Input: part model. Units: mm. Frame: model coordinates. A direction names the side the tool comes from. Coordinates: 2 decimals unless noted, no trailing zeros. Write each loop counter-clockwise with the first axis right and the second up, starting at its lowest first coordinate (ties: lowest second). Pieces come first, ordered by that corner, then holes.
1) Section query D-D (x = -7). Output: boundary loops of the cut face in (y, z).
2) Section query C-C (y = 3.75). Output: boundary loops of the cut face in (x, z).
3) Pin query (flat end, axial travel): pin 1 Ø2.5 at (x, z) = (0, 0) entering from -Y; pin 2 Ø2 at (x, y) = (-7, 1) entering from -Z; pin 3 Ø1.5 at (y, z) = (2.5, 7.5) entering from +X; pin 4 Ø4 at (x, z) = (0, 7) entering from +Y. Return the tip coordinate at first contact, or that it passes through.
4) Section query B-B (z = -7). Output: boundary loops of the cut face in (x, y).
5) Section query A-A (x = 0). Output: boundary loops of the cut face in (y, z).
6) Set-up query: faces 4 (the cylindrical face through (5.536, 0.986, -0.325)), 5 (the flat face through (-2.1, 2, 4.3)). Return all of +Z, -Z, +X, -X, +Y, -Y with unobstructed straight access to the full face (end or side cutting, diameter ignored); none if empty.
7) Draft query along Z for faces 1 (the cylindrical face through (-8.464, 0.986, -0.325)), 2 (the cylindrical face through (-9.76, 0.99, -2.17)), 3 (the flat face through (-2, 4.5, 2)). Return one class per face: pulls with the +Z half, pulls with the -Z half, needs draft (parallel to the pull), parting line crosses it, or undercut.
8) Line query: L1, parallel to X at y = 0.55, z = 0; L2, parallel to X at y = 1.25, z = 0; L3, parallel to Y at x = -9, z = -0.25. Output: solid intervals per line, ascending.
from build123d import *

# Parameters (mm, degrees)
SKETCH_1_R          = 10
SKETCH_1_R_2        = 1.5
EXTRUDE_1_DEPTH     = 2
SKETCH_2_R          = 4.5
EXTRUDE_2_DEPTH     = 2.5
SKETCH_3_R          = 1.5
CUT_EXTRUDE_1_DEPTH = 15.84082208
SKETCH_4_R          = 2.5
CUT_EXTRUDE_2_DEPTH = 3.5


with BuildPart() as part:
    # 草图1 → 凸台-拉伸1 (new body)
    with BuildSketch(Plane(origin=(0, 0, 0), x_dir=(1, 0, 0), z_dir=(0, 1, 0))):
        with Locations(Location((0, 0, 0), (0, 0, 270))):
            Circle(SKETCH_1_R)
        with Locations(Location((0, 7, 0), (0, 0, 270))):
            Circle(SKETCH_1_R_2, mode=Mode.SUBTRACT)
        with Locations(Location((7, 0, 0), (0, 0, 270))):
            Circle(SKETCH_1_R_2, mode=Mode.SUBTRACT)
        with Locations(Location((0, -7, 0), (0, 0, 270))):
            Circle(SKETCH_1_R_2, mode=Mode.SUBTRACT)
        with Locations(Location((-7, 0, 0), (0, 0, 270))):
            Circle(SKETCH_1_R_2, mode=Mode.SUBTRACT)
    extrude(amount=EXTRUDE_1_DEPTH)

    # 草图2 → 凸台-拉伸2 (add)
    with BuildSketch(Plane(origin=(0, 2, 0), x_dir=(1, 0, 0), z_dir=(0, 1, 0))):
        with Locations(Location((0, 0, 0), (0, 0, 270))):
            Circle(SKETCH_2_R)
    extrude(amount=EXTRUDE_2_DEPTH)

    # 草图3 → 切除-拉伸1 (cut, through all)
    with BuildSketch(Plane(origin=(0, 4.5, 0), x_dir=(1, 0, 0), z_dir=(0, 1, 0))):
        with Locations(Location((0, 0, 0), (0, 0, 270))):
            Circle(SKETCH_3_R)
    extrude(amount=-CUT_EXTRUDE_1_DEPTH, mode=Mode.SUBTRACT)

    # 草图4 → 切除-拉伸2 (cut)
    with BuildSketch(Plane(origin=(0, 4.5, 0), x_dir=(1, 0, 0), z_dir=(0, 1, 0))):
        with Locations(Location((0, 0, 0), (0, 0, 270))):
            Circle(SKETCH_4_R)
    extrude(amount=-CUT_EXTRUDE_2_DEPTH, mode=Mode.SUBTRACT)


solid = part.part
Answer:
1. outline: (0, -7.14) - (2, -7.14) - (2, -1.5) - (0, -1.5) - close; (0, 1.5) - (2, 1.5) - (2, 7.14) - (0, 7.14) - close
2. outline: circle Ø9 at (0, 0); hole circle Ø5 at (0, 0)
3. pin 1: passes through
3. pin 2: stops at z = -8
3. pin 3: stops at x = 7.2
3. pin 4: stops at y = 2
4. outline: (-7.14, 0) - (-1.5, 0) - (-1.5, 2) - (-7.14, 2) - close; (1.5, 0) - (7.14, 0) - (7.14, 2) - (1.5, 2) - close
5. outline: (0, -10) - (2, -10) - (2, -8.5) - (0, -8.5) - close; (0, -5.5) - (2, -5.5) - (2, -4.5) - (4.5, -4.5) - (4.5, -2.5) - (1, -2.5) - (1, -1.5) - (0, -1.5) - close; (0, 1.5) - (1, 1.5) - (1, 2.5) - (4.5, 2.5) - (4.5, 4.5) - (2, 4.5) - (2, 5.5) - (0, 5.5) - close; (0, 8.5) - (2, 8.5) - (2, 10) - (0, 10) - close
6. face 4: +Y, -Y
6. face 5: +Y
7. face 1: undercut
7. face 2: parting line crosses it
7. face 3: needs draft
8. L1: x = -10 to -8.5, -5.5 to -1.5, 1.5 to 5.5, 8.5 to 10
8. L2: x = -10 to -8.5, -5.5 to -2.5, 2.5 to 5.5, 8.5 to 10
8. L3: y = 0 to 2
